```python
from build123d import *

# Parameters (mm, degrees)
SKETCH1_W              = 273.05
SKETCH1_H              = 139.7
BOSS_EXTRUDE1_DEPTH    = 5.588
SKETCH2_W              = 273.05
SKETCH2_H              = 139.7
SKETCH2_W_2            = 261.874
SKETCH2_H_2            = 128.524
BOSS_EXTRUDE2_DEPTH    = 298.45
SKETCH3_W              = 6.35
SKETCH3_H              = 16.933333333
SKETCH3_H_2            = 16.933333334
DOOR_SLOT_DEPTH        = 12.7
DOOR_GUIDE_HOLES_REACH = 361.255
SKETCH4_W              = 6.35
SKETCH4_H              = 15.875
LEVER_HOLES_W          = 9.652
LEVER_HOLES_H          = 6.35
LEVER_HOLES_W_2        = 6.35
CUT_EXTRUDE1_DEPTH     = 362.378293578
CUT_EXTRUDE3_REACH     = 416.577
SKETCH8_R              = 3.175
SKETCH16_W             = 327.238778096
SKETCH16_H             = 314.471565403
CUT_EXTRUDE10_DEPTH    = 362.378293578
LEFT_RIGHT_W           = 6.35
LEFT_RIGHT_H           = 5.588
LEFT_RIGHT_W_2         = 12.7
LEFT_RIGHT_H_2         = 12.66825
CUT_EXTRUDE11_DEPTH    = 415.577411883
SKETCH17_R             = 1.5
SKETCH17_W             = 23
SKETCH17_H             = 17.61800007
CUT_EXTRUDE12_DEPTH    = 313.00857951


with BuildPart() as part:
    # Sketch1 → Boss-Extrude1 (new body)
    with BuildSketch(Plane(origin=(0, 0, 0), x_dir=(1, 0, 0), z_dir=(0, 1, 0))):
        Rectangle(SKETCH1_W, SKETCH1_H)
    extrude(amount=BOSS_EXTRUDE1_DEPTH)

    # Sketch2 → Boss-Extrude2 (add)
    with BuildSketch(Plane(origin=(0, 5.588, 0), x_dir=(1, 0, 0), z_dir=(0, 1, 0))):
        Rectangle(SKETCH2_W, SKETCH2_H)
        Rectangle(SKETCH2_W_2, SKETCH2_H_2, mode=Mode.SUBTRACT)
    extrude(amount=BOSS_EXTRUDE2_DEPTH)

    # Sketch3 → Door Slot (cut)
    with BuildSketch(Plane.XY.offset(69.85)):
        with BuildLine():
            Line((-29.337, 282.448), (-29.337, 5.588))
            Line((-29.337, 5.588), (-22.733, 5.588))
            Line((-22.733, 5.588), (-22.733, 291.592))
            Line((-22.733, 291.592), (-42.291, 291.592))
            Line((-42.291, 291.592), (-42.291, 284.988))
            Line((-42.291, 284.988), (-31.877, 284.988))
            ThreePointArc((-31.877, 284.988), (-30.080948776, 284.244051224), (-29.337, 282.448))
        make_face()
        with Locations((-13.208, 80.433333334)):
            Rectangle(SKETCH3_W, SKETCH3_H)
        with Locations((-13.208, 50.8)):
            Rectangle(SKETCH3_W, SKETCH3_H_2)
        with Locations((-13.208, 21.166666667)):
            Rectangle(SKETCH3_W, SKETCH3_H)
    extrude(amount=-DOOR_SLOT_DEPTH, mode=Mode.SUBTRACT)

    # Sketch4 → Door Guide Holes (cut, up to next)
    with BuildSketch(Plane.XY.offset(-64.262), mode=Mode.PRIVATE) as door_guide_holes_sk1:
        with Locations((-45.466, 283.4005)):
            Rectangle(SKETCH4_W, SKETCH4_H)
    door_guide_holes_tool1 = extrude(door_guide_holes_sk1.sketch, amount=-DOOR_GUIDE_HOLES_REACH, mode=Mode.PRIVATE) & part.part
    # Sketch4 → Door Guide Holes (cut, up to next)
    with BuildSketch(Plane.XY.offset(-64.262), mode=Mode.PRIVATE) as door_guide_holes_sk2:
        with Locations((-45.466, 254.8255)):
            Rectangle(SKETCH4_W, SKETCH4_H)
    door_guide_holes_tool2 = extrude(door_guide_holes_sk2.sketch, amount=-DOOR_GUIDE_HOLES_REACH, mode=Mode.PRIVATE) & part.part
    # Sketch4 → Door Guide Holes (cut, up to next)
    with BuildSketch(Plane.XY.offset(-64.262), mode=Mode.PRIVATE) as door_guide_holes_sk3:
        with Locations((-45.466, 226.2505)):
            Rectangle(SKETCH4_W, SKETCH4_H)
    door_guide_holes_tool3 = extrude(door_guide_holes_sk3.sketch, amount=-DOOR_GUIDE_HOLES_REACH, mode=Mode.PRIVATE) & part.part
    # Sketch4 → Door Guide Holes (cut, up to next)
    with BuildSketch(Plane.XY.offset(-64.262), mode=Mode.PRIVATE) as door_guide_holes_sk4:
        with Locations((-45.466, 197.6755)):
            Rectangle(SKETCH4_W, SKETCH4_H)
    door_guide_holes_tool4 = extrude(door_guide_holes_sk4.sketch, amount=-DOOR_GUIDE_HOLES_REACH, mode=Mode.PRIVATE) & part.part
    # Sketch4 → Door Guide Holes (cut, up to next)
    with BuildSketch(Plane.XY.offset(-64.262), mode=Mode.PRIVATE) as door_guide_holes_sk5:
        with Locations((-45.466, 169.1005)):
            Rectangle(SKETCH4_W, SKETCH4_H)
    door_guide_holes_tool5 = extrude(door_guide_holes_sk5.sketch, amount=-DOOR_GUIDE_HOLES_REACH, mode=Mode.PRIVATE) & part.part
    # Sketch4 → Door Guide Holes (cut, up to next)
    with BuildSketch(Plane.XY.offset(-64.262), mode=Mode.PRIVATE) as door_guide_holes_sk6:
        with Locations((-45.466, 140.5255)):
            Rectangle(SKETCH4_W, SKETCH4_H)
    door_guide_holes_tool6 = extrude(door_guide_holes_sk6.sketch, amount=-DOOR_GUIDE_HOLES_REACH, mode=Mode.PRIVATE) & part.part
    # Sketch4 → Door Guide Holes (cut, up to next)
    with BuildSketch(Plane.XY.offset(-64.262), mode=Mode.PRIVATE) as door_guide_holes_sk7:
        with Locations((-45.466, 111.9505)):
            Rectangle(SKETCH4_W, SKETCH4_H)
    door_guide_holes_tool7 = extrude(door_guide_holes_sk7.sketch, amount=-DOOR_GUIDE_HOLES_REACH, mode=Mode.PRIVATE) & part.part
    # Sketch4 → Door Guide Holes (cut, up to next)
    with BuildSketch(Plane.XY.offset(-64.262), mode=Mode.PRIVATE) as door_guide_holes_sk8:
        with Locations((-45.466, 83.3755)):
            Rectangle(SKETCH4_W, SKETCH4_H)
    door_guide_holes_tool8 = extrude(door_guide_holes_sk8.sketch, amount=-DOOR_GUIDE_HOLES_REACH, mode=Mode.PRIVATE) & part.part
    # Sketch4 → Door Guide Holes (cut, up to next)
    with BuildSketch(Plane.XY.offset(-64.262), mode=Mode.PRIVATE) as door_guide_holes_sk9:
        with Locations((-45.466, 54.8005)):
            Rectangle(SKETCH4_W, SKETCH4_H)
    door_guide_holes_tool9 = extrude(door_guide_holes_sk9.sketch, amount=-DOOR_GUIDE_HOLES_REACH, mode=Mode.PRIVATE) & part.part
    # Sketch4 → Door Guide Holes (cut, up to next)
    with BuildSketch(Plane.XY.offset(-64.262), mode=Mode.PRIVATE) as door_guide_holes_sk10:
        with Locations((-45.466, 26.2255)):
            Rectangle(SKETCH4_W, SKETCH4_H)
    door_guide_holes_tool10 = extrude(door_guide_holes_sk10.sketch, amount=-DOOR_GUIDE_HOLES_REACH, mode=Mode.PRIVATE) & part.part
    door_guide_holes_1 = door_guide_holes_tool1.solids().sort_by_distance((-45.466, 283.4005, -64.262))[0]
    add(door_guide_holes_1, mode=Mode.SUBTRACT)
    door_guide_holes_2 = door_guide_holes_tool2.solids().sort_by_distance((-45.466, 254.8255, -64.262))[0]
    add(door_guide_holes_2, mode=Mode.SUBTRACT)
    door_guide_holes_3 = door_guide_holes_tool3.solids().sort_by_distance((-45.466, 226.2505, -64.262))[0]
    add(door_guide_holes_3, mode=Mode.SUBTRACT)
    door_guide_holes_4 = door_guide_holes_tool4.solids().sort_by_distance((-45.466, 197.6755, -64.262))[0]
    add(door_guide_holes_4, mode=Mode.SUBTRACT)
    door_guide_holes_5 = door_guide_holes_tool5.solids().sort_by_distance((-45.466, 169.1005, -64.262))[0]
    add(door_guide_holes_5, mode=Mode.SUBTRACT)
    door_guide_holes_6 = door_guide_holes_tool6.solids().sort_by_distance((-45.466, 140.5255, -64.262))[0]
    add(door_guide_holes_6, mode=Mode.SUBTRACT)
    door_guide_holes_7 = door_guide_holes_tool7.solids().sort_by_distance((-45.466, 111.9505, -64.262))[0]
    add(door_guide_holes_7, mode=Mode.SUBTRACT)
    door_guide_holes_8 = door_guide_holes_tool8.solids().sort_by_distance((-45.466, 83.3755, -64.262))[0]
    add(door_guide_holes_8, mode=Mode.SUBTRACT)
    door_guide_holes_9 = door_guide_holes_tool9.solids().sort_by_distance((-45.466, 54.8005, -64.262))[0]
    add(door_guide_holes_9, mode=Mode.SUBTRACT)
    door_guide_holes_10 = door_guide_holes_tool10.solids().sort_by_distance((-45.466, 26.2255, -64.262))[0]
    add(door_guide_holes_10, mode=Mode.SUBTRACT)
    door_guide_holes = door_guide_holes_1 + door_guide_holes_2 + door_guide_holes_3 + door_guide_holes_4 + door_guide_holes_5 + door_guide_holes_6 + door_guide_holes_7 + door_guide_holes_8 + door_guide_holes_9 + door_guide_holes_10  # Door Guide Holes as one shape, for the pattern or mirror that repeats it

    # Mirror1: Door Guide Holes across plane
    add(door_guide_holes.mirror(Plane.ZY.offset(32.512)), mode=Mode.SUBTRACT)

    # Lever Holes → Cut-Extrude1 (cut, through all)
    with BuildSketch(Plane.XY.offset(69.85)):
        with Locations((54.102, 28.575)):
            Rectangle(LEVER_HOLES_W, LEVER_HOLES_H)
        with Locations((39.3065, 15.875)):
            Rectangle(LEVER_HOLES_W_2, LEVER_HOLES_H)
        with Locations((68.8975, 15.875)):
            Rectangle(LEVER_HOLES_W_2, LEVER_HOLES_H)
    extrude(amount=-CUT_EXTRUDE1_DEPTH, mode=Mode.SUBTRACT)

    # Sketch8 → Cut-Extrude3 (cut, up to next)
    with BuildSketch(Plane.ZY.offset(136.525), mode=Mode.PRIVATE) as cut_extrude3_sk1:
        with Locations((0, 19.05)):
            Circle(SKETCH8_R)
    cut_extrude3_tool1 = extrude(cut_extrude3_sk1.sketch, amount=-CUT_EXTRUDE3_REACH, mode=Mode.PRIVATE) & part.part
    add(cut_extrude3_tool1.solids().sort_by_distance((-136.525, 19.05, 0))[0], mode=Mode.SUBTRACT)

    # Sketch16 → Cut-Extrude10 (cut, through all)
    with BuildSketch(Plane.XY.offset(69.85)):
        with Locations((-32.682389048, 146.802217299)):
            Rectangle(SKETCH16_W, SKETCH16_H)
    extrude(amount=-CUT_EXTRUDE10_DEPTH, mode=Mode.SUBTRACT)

    # Left/Right → Cut-Extrude11 (cut, through all)
    with BuildSketch(Plane.ZY.offset(136.525)):
        with Locations((60.325, 2.794)):
            Rectangle(LEFT_RIGHT_W, LEFT_RIGHT_H)
        with Locations((38.1, 2.794)):
            Rectangle(LEFT_RIGHT_W_2, LEFT_RIGHT_H)
        with Locations((66.675, 19.002375)):
            Rectangle(LEFT_RIGHT_W, LEFT_RIGHT_H_2)
        with Locations((12.7, 2.794)):
            Rectangle(LEFT_RIGHT_W_2, LEFT_RIGHT_H)
        with Locations((66.675, 44.338875)):
            Rectangle(LEFT_RIGHT_W, LEFT_RIGHT_H_2)
        with Locations((-12.7, 2.794)):
            Rectangle(LEFT_RIGHT_W_2, LEFT_RIGHT_H)
        with Locations((66.675, 69.675375)):
            Rectangle(LEFT_RIGHT_W, LEFT_RIGHT_H_2)
        with Locations((-38.1, 2.794)):
            Rectangle(LEFT_RIGHT_W_2, LEFT_RIGHT_H)
        with Locations((66.675, 95.011875)):
            Rectangle(LEFT_RIGHT_W, LEFT_RIGHT_H_2)
        with Locations((-60.325, 2.794)):
            Rectangle(LEFT_RIGHT_W, LEFT_RIGHT_H)
        with Locations((66.675, 120.348375)):
            Rectangle(LEFT_RIGHT_W, LEFT_RIGHT_H_2)
        with Locations((-66.675, 19.002375)):
            Rectangle(LEFT_RIGHT_W, LEFT_RIGHT_H_2)
        with Locations((66.675, 145.684875)):
            Rectangle(LEFT_RIGHT_W, LEFT_RIGHT_H_2)
        with Locations((-66.675, 44.338875)):
            Rectangle(LEFT_RIGHT_W, LEFT_RIGHT_H_2)
        with Locations((66.675, 171.021375)):
            Rectangle(LEFT_RIGHT_W, LEFT_RIGHT_H_2)
        with Locations((-66.675, 69.675375)):
            Rectangle(LEFT_RIGHT_W, LEFT_RIGHT_H_2)
        with Locations((66.675, 196.357875)):
            Rectangle(LEFT_RIGHT_W, LEFT_RIGHT_H_2)
        with Locations((-66.675, 95.011875)):
            Rectangle(LEFT_RIGHT_W, LEFT_RIGHT_H_2)
        with Locations((66.675, 221.694375)):
            Rectangle(LEFT_RIGHT_W, LEFT_RIGHT_H_2)
        with Locations((-66.675, 120.348375)):
            Rectangle(LEFT_RIGHT_W, LEFT_RIGHT_H_2)
        with Locations((66.675, 247.030875)):
            Rectangle(LEFT_RIGHT_W, LEFT_RIGHT_H_2)
        with Locations((-66.675, 145.684875)):
            Rectangle(LEFT_RIGHT_W, LEFT_RIGHT_H_2)
        with Locations((66.675, 272.367375)):
            Rectangle(LEFT_RIGHT_W, LEFT_RIGHT_H_2)
        with Locations((-66.675, 171.021375)):
            Rectangle(LEFT_RIGHT_W, LEFT_RIGHT_H_2)
        with Locations((66.675, 297.703875)):
            Rectangle(LEFT_RIGHT_W, LEFT_RIGHT_H_2)
        with Locations((-66.675, 196.357875)):
            Rectangle(LEFT_RIGHT_W, LEFT_RIGHT_H_2)
        with Locations((-66.675, 221.694375)):
            Rectangle(LEFT_RIGHT_W, LEFT_RIGHT_H_2)
        with Locations((-66.675, 247.030875)):
            Rectangle(LEFT_RIGHT_W, LEFT_RIGHT_H_2)
        with Locations((-66.675, 272.367375)):
            Rectangle(LEFT_RIGHT_W, LEFT_RIGHT_H_2)
        with Locations((-66.675, 297.703875)):
            Rectangle(LEFT_RIGHT_W, LEFT_RIGHT_H_2)
    extrude(amount=-CUT_EXTRUDE11_DEPTH, mode=Mode.SUBTRACT)

    # Sketch17 → Cut-Extrude12 (cut, through all)
    with BuildSketch(Plane(origin=(136.525, 0, 0), x_dir=(0, 0, -1), z_dir=(1, 0, 0))):
        with Locations((-8, 62.088)):
            Circle(SKETCH17_R)
        with Locations((8, 62.088)):
            Circle(SKETCH17_R)
        with Locations((-50.8, 159.894)):
            Circle(SKETCH17_R)
        with Locations((-50.8, 144.144)):
            Circle(SKETCH17_R)
        with Locations(Location((50.8, 144.144, 0), (0, 0, 180))):
            Circle(SKETCH17_R)
        with Locations(Location((50.8, 159.894, 0), (0, 0, 180))):
            Circle(SKETCH17_R)
        with Locations((0, 22.779000035)):
            Rectangle(SKETCH17_W, SKETCH17_H)
    extrude(amount=-CUT_EXTRUDE12_DEPTH, mode=Mode.SUBTRACT)


solid = part.part
```
Source: CAD feature listing. Evaluate the final solid. Frame: model axes, mm. A direction names the side the tool comes from. Round coordinates to 2 decimals unless told otherwise and drop trailing zeros. Order: outer loops, then holes, each group sorted by start corner. A loop starts at its lowest first (then second) coordinate and runs counter-clockwise, first axis right, second up. Notation, with made-up numbers: (-29, 23) -> (3, 23) arc R20 cw to (3, 29) -> close; hole circle Ø5 at (-18.5, 26.25). An arc over 180 degrees is marked (long way). One line per item, written item: value. Start each with the question number.
Q1. Pin query (flat end, axial travel): pin 1 (1.5 mm diameter, centred on x = 133, z = 13, fed in from -Y); pin 2 (3 mm diameter, centred on x = 134.5, z = -66, fed in from +Y); pin 3 (3 mm diameter, centred on x = 133, y = 92.5, fed in from +Z). Return the tip coordinate at first contact, or that it passes through.
Q2. Access query for faces 1 (the flat face through (134, 3, 6.35)), 2 (the flat face through (134, 215.36, 67)), 3 (the flat face through (134, 0, -51)), 4 (the flat face through (134, 152.019, -67)). Directions: +Z, -Z, +X, -X, +Y, -Y. A direction counts if a zero-diameter tool reaches every point of the face in a straight line with its end or side. Return the directions, or none.
Q3. Draft query along Z for faces 5 (the flat face through (134, 70, -63.5)), 6 (the flat face through (134, 260, 69.85)), 7 (the flat face through (134, 3, -63.5)). Return one class per face: pulls with the +Z half, pulls with the -Z half, needs draft (parallel to the pull), parting line crosses it, or undercut.
Q4. Material intervals for probe 1 along Y at (x, z) = (134.1, 50.8); probe 2 along Z at (x, y) = (132.55, 61.5); probe 3 along Z at (x, y) = (132.4, 198.5), sorted ascending.
Q5. Section query B-B (x = 134.25). Give the number of separate pieces and of enclosed holes in the cut face, plus the area to 3 significant figures.
Q6. Section query A-A (z = -16). Return the cut outline in (x, y) (3 decimals).
Findings below:
1. pin 1: y = 5.59
1. pin 2: y = 291.37
1. pin 3: z = 63.5
2. face 1: +X, -X, -Y
2. face 2: +Z, +X, -X
2. face 3: +Z, -Z, +X, -X, -Y
2. face 4: -Z, +X, -X
3. face 5: pulls with the -Z half
3. face 6: pulls with the +Z half
3. face 7: undercut
4. probe 1: 0 to 142.64, 145.64 to 158.39, 161.39 to 304.04
4. probe 2: -69.85 to -9.38, -6.62 to 6.62, 9.38 to 69.85
4. probe 3: -63.5 to 63.5
5. separate pieces: 1
5. enclosed holes: 7
5. area: 39,700 mm²
6. outline: (130.937, 5.588) -> (136.525, 5.588) -> (136.525, 304.038) -> (130.937, 304.038) -> close
